from build123d import *

# Parameters (mm, degrees)
SKETCH1_R           = 20
BOSS_EXTRUDE1_DEPTH = 8
SKETCH2_R           = 10
BOSS_EXTRUDE2_DEPTH = 17
M12_TAPPED_HOLE1_D  = 10.2
CHAMFER1_SIZE       = 1
M5_TAPPED_HOLE1_D   = 4.2
CUT_EXTRUDE1_REACH  = 39.749
SKETCH7_W           = 49.327328333
SKETCH7_H           = 13.526029649
CHAMFER2_SIZE       = 0.5


with BuildPart() as part:
    # Sketch1 → Boss-Extrude1 (new body)
    with BuildSketch(Plane(origin=(0, 0, 0), x_dir=(1, 0, 0), z_dir=(0, 1, 0))):
        with Locations(Location((0, 0, 0), (0, 0, 270))):
            Circle(SKETCH1_R)
    extrude(amount=BOSS_EXTRUDE1_DEPTH)

    # Sketch2 → Boss-Extrude2 (add)
    with BuildSketch(Plane(origin=(0, 8, 0), x_dir=(1, 0, 0), z_dir=(0, 1, 0))):
        with Locations(Location((0, 0, 0), (0, 0, 270))):
            Circle(SKETCH2_R)
    extrude(amount=BOSS_EXTRUDE2_DEPTH)

    # M12 Tapped Hole1 (through all)
    with Locations(Plane(origin=(0, 25, 0), x_dir=(-1, 0, 0), z_dir=(0, 1, 0))):
        with Locations((0, 0)):
            Hole(M12_TAPPED_HOLE1_D / 2)

    # Chamfer1
    chamfer1_edges = [part.edges().sort_by_distance(p)[0] for p in [
        (-5.1, 25, 0),
        (-5.1, 0, 0),
    ]]
    chamfer(chamfer1_edges, length=CHAMFER1_SIZE)

    # M5 Tapped Hole1 (through all)
    with Locations(Plane(origin=(0, 8, 0), x_dir=(-1, 0, 0), z_dir=(0, 1, 0))):
        with Locations((15, 0), (-15, 0)):
            Hole(M5_TAPPED_HOLE1_D / 2)

    # Sketch7 → Cut-Extrude1 (cut, up to next)
    with BuildSketch(Plane.XZ, mode=Mode.PRIVATE) as cut_extrude1_sk1:
        with Locations((2.087303486, 21.763014825)):
            Rectangle(SKETCH7_W, SKETCH7_H)
    cut_extrude1_tool1 = extrude(cut_extrude1_sk1.sketch, amount=-CUT_EXTRUDE1_REACH, mode=Mode.PRIVATE) & part.part
    add(cut_extrude1_tool1.solids().sort_by_distance((2.087303, 0, 21.763015))[0], mode=Mode.SUBTRACT)

    # Chamfer2
    chamfer2_edges = [part.edges().sort_by_distance(p)[0] for p in [
        (0, 0, -20),
        (0, 8, 15),
        (0, 0, 15),
        (0, 8, -20),
        (0, 25, -10),
    ]]
    chamfer(chamfer2_edges, length=CHAMFER2_SIZE)


solid = part.part
Model file for the job. Use its own axes, mm. A direction names the side the tool comes from. Coordinates: 2 decimals unless noted, no trailing zeros. Loops run counter-clockwise (first coordinate to the right, second up) from the corner with the lowest first, then second, coordinate; pieces in that order, holes last. Notation, with made-up numbers: (-20, 64.25) -> (8, 64.25) arc R27 ccw to (8, 100.25) -> close; hole circle Ø6 at (-9.5, 28.5). An arc over 180 degrees is marked (long way). Use one line per item in the form item = value. Start each with the question number.
(1) Cut at A-A on x = 0. Give the cut face in (y, z).
(2) Cut at D-D on y = 5.5. Give the cut face in (x, z), and give its area (3 significant figures).
(3) Probe probe 1 along Z at (x, y) = (-15, 4.75); probe 2 along Y at (x, z) = (6, -10.5); probe 3 along Z at (x, y) = (3, 4.75). List the from-to ranges inside material, lowest first. Write a range as from..to.
(4) Cut at C-C on y = 20.5. Give the cut face in (x, z).
(5) Flat gauge pins, fed straight in: pin 1 (4 mm diameter, centred on x = 15, z = 0, fed in from -Y); pin 2 (5 mm diameter, centred on x = 7, z = -10.5, fed in from +Y); pin 3 (1.5 mm diameter, centred on x = 5.5, y = 15, fed in from -Z); pin 4 (3 mm diameter, centred on y = 17, z = 6, fed in from -X). Where does each tip first touch, or does it go through?
(6) Pull direction Z, two halves, no side cores. Call faces 1 (the conical face through (0.665, 7.865, -19.624)), 2 (the flat face through (0, 0, -7)), 3 (the cylindrical face through (2.4, 12.3, -4.5)), 4 (the cylindrical face through (-17.1, 3.94, 0.09)): pulls with the +Z half, pulls with the -Z half, needs draft (parallel to the pull), parting line crosses it, or undercut.
(7) Tool access for faces 5 (the conical face through (0.67, 0.14, -19.63)), 6 (the flat face through (0.3, 8, -10.3)): list every direction of +Z, -Z, +X, -X, +Y, -Y with a clear straight run to the whole face (end or side of a thin tool).
(8) Cut at B-B on z = 0. Give the number of separate pieces and of enclosed holes in the cut face, and give its area (3 significant figures).
Values:
q1.outline = (0, -19.5) -> (0.5, -20) -> (7.5, -20) -> (8, -19.5) -> (8, -10) -> (24.5, -10) -> (25, -9.5) -> (25, -6.1) -> (24, -5.1) -> (1, -5.1) -> (0, -6.1) -> close; (0, 6.1) -> (1, 5.1) -> (24, 5.1) -> (25, 6.1) -> (25, 9.5) -> (24.5, 10) -> (8, 10) -> (8, 14.5) -> (7.5, 15) -> (0.5, 15) -> (0, 14.5) -> close
q2.outline = (-13.23, 15) arc R20 ccw (long way) to (13.23, 15) -> close; hole circle Ø4.2 at (-15, 0); hole circle Ø10.2 at (0, 0); hole circle Ø4.2 at (15, 0)
q2.area = 1,060 mm2
q3.probe_1 = -13.23..-2.1, 2.1..13.23
q3.probe_2 = 0..8
q3.probe_3 = -19.77..-4.12, 4.12..15
q4.outline = circle Ø20 at (0, 0); hole circle Ø10.2 at (0, 0)
q5.pin_1 = through
q5.pin_2 = 8
q5.pin_3 = -8.8
q5.pin_4 = -8.93
q6.face_1 = parting line crosses it
q6.face_2 = needs draft
q6.face_3 = undercut
q6.face_4 = undercut
q7.face_5 = -Y
q7.face_6 = +Y
q8.separate_pieces = 4
q8.enclosed_holes = 0
q8.area = 335 mm2
